Work out the finished part from the listing and answer in its coordinate system (mm). Face numbers are marked on the shaded views. Give positions to 0.01 mm unless a question says otherwise; leave off trailing zeros. Order: outer loops, then holes, each group sorted by start corner. A loop starts at its lowest first (then second) coordinate and runs counter-clockwise, first axis right, second up. Notation, with made-up numbers: (-30.5, 81.25) - (13.5, 81.25) arc R15 cw to (13.5, 104.25) - close; hole circle Ø4 at (29.5, -3.5). An arc over 180 degrees is marked (long way). Put each result on its own line as item: value.
```python
from build123d import *

# Parameters (mm, degrees)
SKETCH_W            = 30
SKETCH_H            = 23
PAD002_DEPTH        = 8
POCKET001_DEPTH     = 1.2
SKETCH002_W         = 0.3
SKETCH002_H         = 23
POCKET_DEPTH        = 1
LINEARPATTERN_COUNT = 9
LINEARPATTERN_PITCH = 2.375


with BuildPart() as part:
    # Sketch → Pad002 (new body)
    with BuildSketch(Plane.XY):
        with Locations((15, 11.5)):
            Rectangle(SKETCH_W, SKETCH_H)
    extrude(amount=PAD002_DEPTH)

    # Sketch001 → Pocket001 (cut)
    with BuildSketch(Plane.XY):
        with BuildLine():
            ThreePointArc((17.966363, 19.215428), (14.961232, 19.999875), (11.966488, 19.17666))
            Line((11.966488, 19.17666), (4.036475, 13.531422))
            ThreePointArc((4.036475, 13.531422), (3.750333, 12.536475), (4, 11.531754))
            Line((4, 11.531754), (12.33, 5.376817))
            ThreePointArc((12.33, 5.376817), (15.374304, 4.761687), (18.318313, 5.75112))
            Line((18.318313, 5.75112), (26, 11.531754))
            ThreePointArc((26, 11.531754), (26.249667, 12.536475), (25.963525, 13.531422))
            Line((25.963525, 13.531422), (17.966363, 19.215428))
        make_face()
    extrude(amount=POCKET001_DEPTH, mode=Mode.SUBTRACT)

    # Sketch002 → Pocket (cut)
    with BuildSketch(Plane.XY):
        with Locations((6.15, 11.5)):
            Rectangle(SKETCH002_W, SKETCH002_H)
    pocket = extrude(amount=POCKET_DEPTH, mode=Mode.SUBTRACT)

    # LinearPattern: Pocket ×9
    with Locations(*[(i * LINEARPATTERN_PITCH, 0, 0) for i in range(1, LINEARPATTERN_COUNT)]):
        add(pocket, mode=Mode.SUBTRACT)


solid = part.part
```
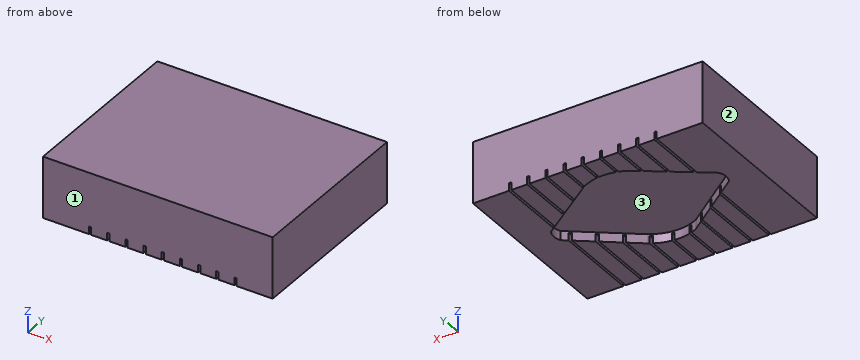
(1) Given pin 1 (5 mm diameter, centred on x = 10, y = 13, fed in from -Z), flat-ended and moving along its own axis, determine where the tip first touches the part or whether it passes through.
Geometry check:
pin 1: stops at z = 1.2
(2) Determine the mould class of the marked faces 1, 2 and 3 for opening direction X: pulls with the +X half, pulls with the -X half, needs draft (parallel to the pull), parting line crosses it, or undercut.
Geometry check:
face 1: needs draft
face 2: pulls with the -X half
face 3: undercut
(3) Section A-A, the plane x = 10 is taken. Write down the section's boundary in (y, z).
Geometry check:
outline: (0, 0) - (7.1, 0) - (7.1, 1.2) - (17.78, 1.2) - (17.78, 0) - (23, 0) - (23, 8) - (0, 8) - close
(4) Straight lines are drawn through the part: line 1 (Y direction, x = 15.25, z = 0.5); line 2 (Z direction, x = 17, y = 11.25); line 3 (Y direction, x = 6.75, z = 0.5). For each, find the intervals that lie inside material, in ascending order.
Geometry check:
line 1: y = 0 to 4.76, 19.99 to 23
line 2: z = 1.2 to 8
line 3: y = 0 to 9.5, 15.46 to 23
(5) Section B-B, the plane x = 4.75 is taken. Write down the section's boundary in (y, z).
Geometry check:
outline: (0, 0) - (10.98, 0) - (10.98, 1.2) - (14.04, 1.2) - (14.04, 0) - (23, 0) - (23, 8) - (0, 8) - close
